```python
from build123d import *

# Parameters (mm, degrees)
BOSS_EXTRUDE1_DEPTH = 2
SKETCH6_R           = 7.5
CUT_EXTRUDE1_DEPTH  = 2
SKETCH7_W           = 96.175516813
SKETCH7_H           = 15.621463592
CUT_EXTRUDE2_DEPTH  = 2


with BuildPart() as part:
    # Sketch5 → Boss-Extrude1 (new body)
    with BuildSketch(Plane.XY):
        with BuildLine():
            Line((-37.65, 16.64), (37.65, 16.64))
            ThreePointArc((37.65, 16.64), (42.65, 0), (37.65, -16.64))
            Line((37.65, -16.64), (-37.65, -16.64))
            ThreePointArc((-37.65, -16.64), (-42.65, 0), (-37.65, 16.64))
        make_face()
    extrude(amount=BOSS_EXTRUDE1_DEPTH)

    # Sketch6 → Cut-Extrude1 (cut)
    with BuildSketch(Plane.XY.offset(2)):
        with Locations((0, 5.34)):
            Circle(SKETCH6_R)
    extrude(amount=-CUT_EXTRUDE1_DEPTH, mode=Mode.SUBTRACT)

    # Sketch7 → Cut-Extrude2 (cut)
    with BuildSketch(Plane.XY.offset(2)):
        with Locations((0.470526011, -14.821569372)):
            Rectangle(SKETCH7_W, SKETCH7_H)
    extrude(amount=-CUT_EXTRUDE2_DEPTH, mode=Mode.SUBTRACT)


solid = part.part
```
The listing builds one solid part. Answer for the finished solid, in the listing's coordinates (mm). Give positions to 0.01 mm unless a question says otherwise; leave off trailing zeros. Order: outer loops, then holes, each group sorted by start corner. A loop starts at its lowest first (then second) coordinate and runs counter-clockwise, first axis right, second up.
1) Find section B-B on y = 8.25. Write down the section's boundary in (x, z), then the cut area to 3 significant figures.
Reported:
outline: (-41.5, 0) - (-6.91, 0) - (-6.91, 2) - (-41.5, 2) - close; (6.91, 0) - (41.5, 0) - (41.5, 2) - (6.91, 2) - close
area: 138 mm2
2) Given P1, Ø5, axis at x = -17.5, y = 13, coming from the -Z side, flat-ended and moving along its own axis, determine where the tip first touches the part or whether it passes through.
Reported:
P1: stops at z = 0
3) Find section C-C on z = 0.65. Write down the section's boundary in (x, y).
Reported:
outline: (-41.82, -7.01) - (41.82, -7.01) arc R30.19 ccw to (37.65, 16.64) - (-37.65, 16.64) arc R30.19 ccw to start; hole circle Ø15 at (0, 5.34)
4) Determine the mould class of faces 1 (the face through (-1, 16.64, 1)), 2 (the face through (-1.63, -1.98, 1.01)), 3 (the face through (-1, -7.011, 1)), 4 (the face through (1, -3, 2)) for opening direction Y: pulls with the +Y half, pulls with the -Y half, needs draft (parallel to the pull), parting line crosses it, or undercut.
Reported:
face 1: pulls with the +Y half
face 2: undercut
face 3: pulls with the -Y half
face 4: needs draft
5) Find section D-D on y = 13.75. Write down the section's boundary in (x, z), then the cut area to 3 significant figures.
Reported:
outline: (-39.34, 0) - (39.34, 0) - (39.34, 2) - (-39.34, 2) - close
area: 157 mm2
6) Consider line 1 along Y through (x, z) = (0, 1.15); line 2 along X through (y, z) = (11.75, 0.9); line 3 along Y through (x, z) = (-3, 0.15). Determine where each line is inside the solid, lowest interval first.
Reported:
line 1: y = -7.01 to -2.16, 12.84 to 16.64
line 2: x = -40.27 to -3.89, 3.89 to 40.27
line 3: y = -7.01 to -1.53, 12.21 to 16.64
7) Find section A-A on x = 0. Write down the section's boundary in (y, z).
Reported:
outline: (-7.01, 0) - (-2.16, 0) - (-2.16, 2) - (-7.01, 2) - close; (12.84, 0) - (16.64, 0) - (16.64, 2) - (12.84, 2) - close
